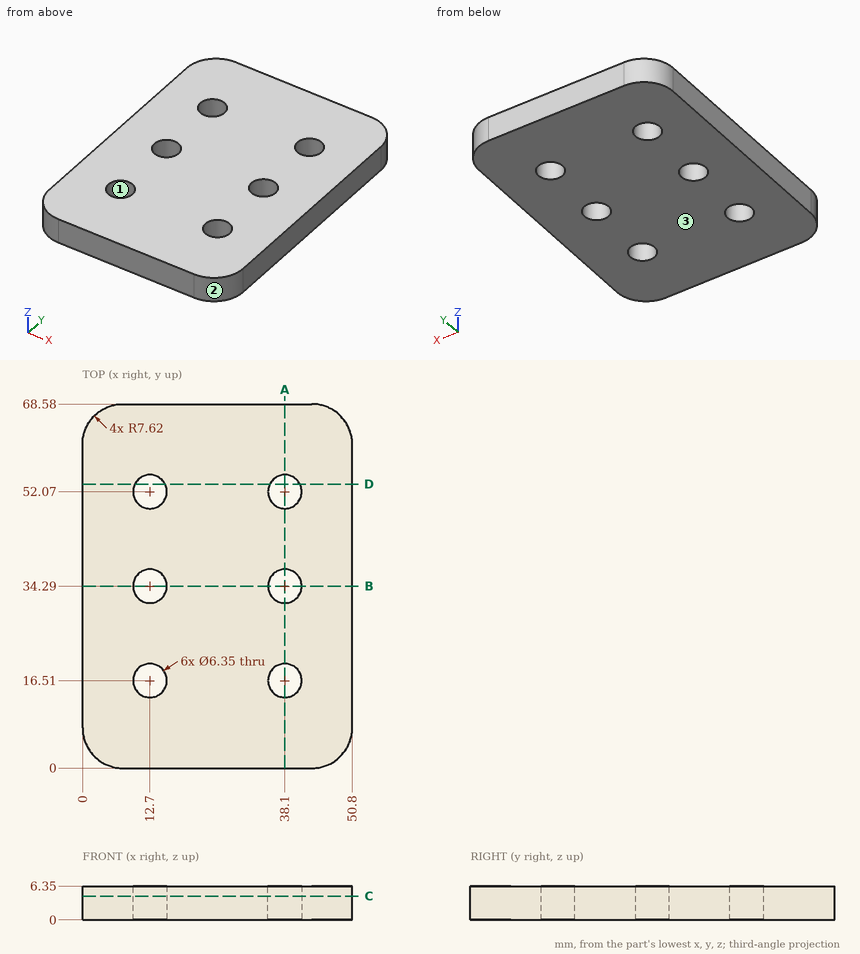
The figure shows three views and two pictorial views of one solid part (mm, origin at its lowest corner). Answer the questions. Round coordinates to 2 decimals unless told otherwise and drop trailing zeros. Order: outer loops, then holes, each group sorted by start corner. A loop starts at its lowest first (then second) coordinate and runs counter-clockwise, first axis right, second up. Notation, with made-up numbers: (87, 82) -> (103, 82) arc R30 cw to (103, 116) -> close; hole circle Ø10 at (22, -16). An arc over 180 degrees is marked (long way). Put each result on its own line as item: value.
Q1. Consider line 1 along Y through (x, z) = (12.7, 1.5) (3 decimals); line 2 along X through (y, z) = (14.5, 2.75); line 3 along Y through (x, z) = (11, 3). Determine where each line is inside the solid, lowest interval first.
Results list:
line 1: 0 to 13.335, 19.685 to 31.115, 37.465 to 48.895, 55.245 to 68.58
line 2: 0 to 10.24, 15.16 to 35.64, 40.56 to 50.8
line 3: 0 to 13.83, 19.19 to 31.61, 36.97 to 49.39, 54.75 to 68.58
Q2. Section B-B, the plane y = 34.29 is taken. Write down the section's boundary in (x, z) (3 decimals), and give its area (3 significant figures).
Results list:
outline: (0, 0) -> (9.525, 0) -> (9.525, 6.35) -> (0, 6.35) -> close; (15.875, 0) -> (34.925, 0) -> (34.925, 6.35) -> (15.875, 6.35) -> close; (41.275, 0) -> (50.8, 0) -> (50.8, 6.35) -> (41.275, 6.35) -> close
area: 242 mm^2
Q3. Section A-A, the plane x = 38.1 is taken. Write down the section's boundary in (y, z) (3 decimals).
Results list:
outline: (0, 0) -> (13.335, 0) -> (13.335, 6.35) -> (0, 6.35) -> close; (19.685, 0) -> (31.115, 0) -> (31.115, 6.35) -> (19.685, 6.35) -> close; (37.465, 0) -> (48.895, 0) -> (48.895, 6.35) -> (37.465, 6.35) -> close; (55.245, 0) -> (68.58, 0) -> (68.58, 6.35) -> (55.245, 6.35) -> close
Q4. Each of these flat-tipped pins is pushed along its axis until it touches: P1, Ø3, axis at x = 25, y = 41, coming from the -Z side; P2, Ø4, axis at x = 12.7, y = 52.07, coming from the +Z side. Where does it stop, or does it pass through?
Results list:
P1: z = 0
P2: through
Q5. Determine the mould class of the marked faces 1, 2 and 3 for opening direction Y: pulls with the +Y half, pulls with the -Y half, needs draft (parallel to the pull), parting line crosses it, or undercut.
Results list:
face 1: undercut
face 2: pulls with the -Y half
face 3: needs draft
Q6. Section C-C, the plane z = 4.5 is taken. Write down the section's boundary in (x, y) (3 decimals).
Results list:
outline: (0, 7.62) arc R7.62 ccw to (7.62, 0) -> (43.18, 0) arc R7.62 ccw to (50.8, 7.62) -> (50.8, 60.96) arc R7.62 ccw to (43.18, 68.58) -> (7.62, 68.58) arc R7.62 ccw to (0, 60.96) -> close; hole circle Ø6.35 at (12.7, 16.51); hole circle Ø6.35 at (12.7, 34.29); hole circle Ø6.35 at (12.7, 52.07); hole circle Ø6.35 at (38.1, 16.51); hole circle Ø6.35 at (38.1, 34.29); hole circle Ø6.35 at (38.1, 52.07)
Q7. Section D-D, the plane y = 53.5 is taken. Write down the section's boundary in (x, z).
Results list:
outline: (0, 0) -> (9.87, 0) -> (9.87, 6.35) -> (0, 6.35) -> close; (15.53, 0) -> (35.27, 0) -> (35.27, 6.35) -> (15.53, 6.35) -> close; (40.93, 0) -> (50.8, 0) -> (50.8, 6.35) -> (40.93, 6.35) -> close
